Can you work these out from the model? Positions are in its coordinate system, mm. Give positions to 0.01 mm unless a question says otherwise; leave off trailing zeros. Loops run counter-clockwise (first coordinate to the right, second up) from the corner with the lowest first, then second, coordinate; pieces in that order, holes last.
Autodesk Inventor part; units mm, degrees
ref_plane "YZ Plane" through (0, 0, 0) normal (1, 0, 0) x (0, 1, 0)
ref_plane "XZ Plane" through (0, 0, 0) normal (0, 1, 0) x (-1, 0, 0)
ref_plane "XY Plane" through (0, 0, 0) normal (0, 0, 1) x (1, 0, 0)
sketch "Szkic6" plane through (0, 0, 0) normal (0, 0, 1) x (1, 0, 0)
  circle A0 centre (-40, -42) radius 2
  circle A1 centre (-40, -8) radius 2
  circle A2 centre (-6, -8) radius 2
  circle A3 centre (-6, -42) radius 2
  circle A4 centre (-23, -25) radius 15
  line L0 (0, -50) -> (0, 0)
  line L1 (-50, 0) -> (0, 0)
  line L2 (-65, -50) -> (-50, 0)
  line L3 (-23, -25) -> (-23, -50)
  line L4 (-23, -50) -> (0, -50)
  line L5 (-23, -50) -> (-65, -50)
  dimension "d30" = 25
extrude "Wyciągnięcie proste4" add sketch "Szkic6" along normal blind 14
properties part number "Wspornik łożyska osi Y - prawa strona"
(1) Suppose I cut it at A-A on y = -37. List the corners of the cut face in (x, z) for me, plus the area to 3 significant figures.
Returned:
outline: (-61.1, 0) - (-32, 0) - (-32, 14) - (-61.1, 14) - close; (-14, 0) - (0, 0) - (0, 14) - (-14, 14) - close
area: 603 mm2
(2) Thinking about a two-plate mould opening in X: for faces 1 (the flat face through (0, -25, 7)), 2 (the cylindrical face through (-6, -40, 7)), 3 (the flat face through (-25, 0, 7)), which applies, pulls with the +X half, pulls with the -X half, needs draft (parallel to the pull), parting line crosses it, or undercut?
Returned:
face 1: pulls with the +X half
face 2: undercut
face 3: needs draft
(3) Please list where these lines run through material, in increasing order: probe 1 along Y at (x, z) = (-6, 10.5); probe 2 along X at (y, z) = (-41.5, 13); probe 3 along Y at (x, z) = (-40.5, 5).
Returned:
probe 1: y = -50 to -44, -40 to -10, -6 to 0
probe 2: x = -62.45 to -41.94, -38.06 to -7.94, -4.06 to 0
probe 3: y = -50 to -43.94, -40.06 to -9.94, -6.06 to 0
(4) Suppose I cut it at C-C on z = 12. List the corners of the cut face in (x, y) for me, plus the area to 3 significant figures.
Returned:
outline: (-65, -50) - (0, -50) - (0, 0) - (-50, 0) - close; hole circle Ø4 at (-40, -42); hole circle Ø4 at (-40, -8); hole circle Ø30 at (-23, -25); hole circle Ø4 at (-6, -42); hole circle Ø4 at (-6, -8)
area: 2,120 mm2
(5) Suppose I cut it at B-B on x = -23. List the corners of the cut face in (y, z) for me, plus the area to 3 significant figures.
Returned:
outline: (-50, 0) - (-40, 0) - (-40, 14) - (-50, 14) - close; (-10, 0) - (0, 0) - (0, 14) - (-10, 14) - close
area: 280 mm2
(6) Will these pins go through, and if not, where does the flat tip stop? P1, Ø2.5, axis at x = -6, y = -8, coming from the +Z side; P2, Ø1.5, axis at y = -12, z = 5, coming from the -X side (3 decimals).
Returned:
P1: passes through
P2: stops at x = -53.825
(7) Suppose I cut it at D-D on x = -6. List the corners of the cut face in (y, z) for me.
Returned:
outline: (-50, 0) - (-44, 0) - (-44, 14) - (-50, 14) - close; (-40, 0) - (-10, 0) - (-10, 14) - (-40, 14) - close; (-6, 0) - (0, 0) - (0, 14) - (-6, 14) - close
